Autodesk Inventor part; units mm, degrees
sketch "Sketch1" plane through (0, 0, 0) normal (0, 1, 0) x (-1, 0, 0)
  line L0 (37.5, 150) -> (-37.5, 150)
  line L1 (-37.5, 150) -> (-37.5, -150)
  line L2 (-37.5, -150) -> (37.5, -150)
  line L3 (37.5, -150) -> (37.5, 150)
  line L4 (37.5, 150) -> (-37.5, -150) construction
  line L5 (-37.5, 150) -> (37.5, -150) construction
  point P0 (0, 0)
  dimension "d0" = 75
  dimension "d1" = 300
extrude "Extrusion1" add sketch "Sketch1" along normal blind 15
sketch "Sketch2" plane through (0, 15, 0) normal (0, 1, 0) x (1, 0, 0)
  line L0 (37.5, -150) -> (37.5, 150)
  line L1 (37.5, 150) -> (-37.5, 150)
  point P0 (0, 0)
  point P1 (22.5, 100)
  dimension "d11" = 15
  dimension "d12" = 50
hole "Hole1" at (22.5, 15, -100) direction (0, -1, 0) diameter 5 end through all
pattern_linear "Rectangular Pattern1" count 2 spacing 50 along (0, 0, 1) of "Hole1"
pattern_linear "Rectangular Pattern2" count 2 spacing 75 along (0, 0, 1) of "Hole1"
pattern_linear "Rectangular Pattern3" count 2 spacing 100 along (0, 0, 1) of "Hole1", "Rectangular Pattern2"
properties part number "PrinterHeadLip_RightSide"
Input: part model. Units: mm. Frame: model coordinates. Round coordinates to 2 decimals unless told otherwise and drop trailing zeros. Write each loop counter-clockwise with the first axis right and the second up, starting at its lowest first coordinate (ties: lowest second). Pieces come first, ordered by that corner, then holes. Notation, with made-up numbers: (44, 76.5) -> (85, 76.5) arc R26 ccw to (85, 111.5) -> close; hole circle Ø4 at (18.5, 7). An arc over 180 degrees is marked (long way). Answer as CSV lines item,"result".
1. Ray query, L1, parallel to Z at x = 22.5, y = 7.5; L2, parallel to X at y = 4, z = -100. Return the intervals inside material, ascending. Write a range as [from, to].
Geometry says:
L1,"z = [-150, -102.5], [-97.5, -52.5], [-47.5, -27.5], [-22.5, -2.5], [2.5, 72.5], [77.5, 150]"
L2,"x = [-37.5, 20], [25, 37.5]"
2. Section A-A (x = 22.5). Return the cut outline in (y, z).
Geometry says:
outline,"(0, -150) -> (15, -150) -> (15, -102.5) -> (0, -102.5) -> close; (0, -97.5) -> (15, -97.5) -> (15, -52.5) -> (0, -52.5) -> close; (0, -47.5) -> (15, -47.5) -> (15, -27.5) -> (0, -27.5) -> close; (0, -22.5) -> (15, -22.5) -> (15, -2.5) -> (0, -2.5) -> close; (0, 2.5) -> (15, 2.5) -> (15, 72.5) -> (0, 72.5) -> close; (0, 77.5) -> (15, 77.5) -> (15, 150) -> (0, 150) -> close"
3. Contact query for a flat-ended pin moving along its axis: P1, Ø6, axis at x = 22.5, z = 75, coming from the +Y side. Output: stop coordinate, or through.
Geometry says:
P1,"stops at y = 15"
4. Section B-B (z = -100). Return the cut outline in (x, y), plus the area to 3 significant figures.
Geometry says:
outline,"(-37.5, 0) -> (20, 0) -> (20, 15) -> (-37.5, 15) -> close; (25, 0) -> (37.5, 0) -> (37.5, 15) -> (25, 15) -> close"
area,"1,050 mm^2"
